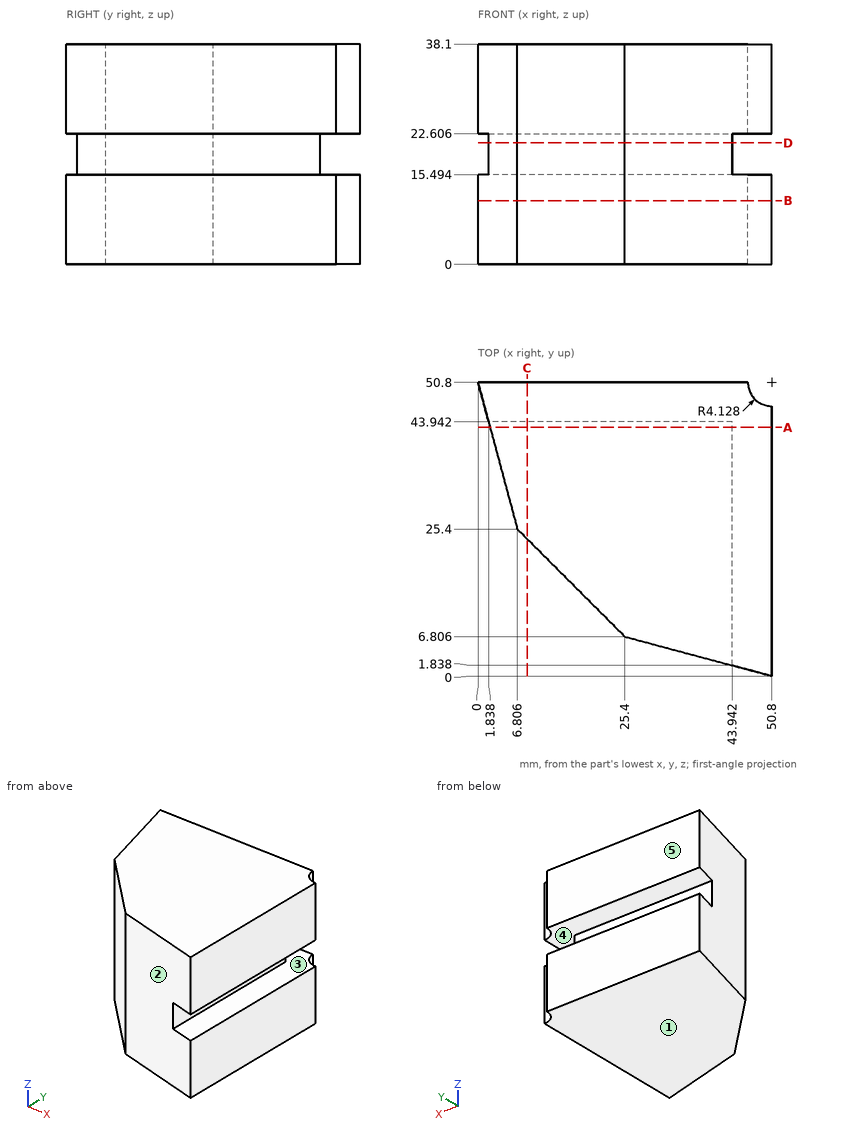
Job drawing, mm, ordinate dimensions from the low corner. One solid piece. A direction names the side the tool comes from. Round coordinates to 2 decimals unless told otherwise and drop trailing zeros. Loops run counter-clockwise (first coordinate to the right, second up) from the corner with the lowest first, then second, coordinate; pieces in that order, holes last. Notation, with made-up numbers: (13, 61) -> (21, 61) arc R11 ccw to (21, 76) -> close; hole circle Ø2 at (-15.75, 49). An arc over 180 degrees is marked (long way). Use CSV: the item, a comma, the result in double quotes. Start each with the question number.
Q1. Saw through at C-C on x = 8.5. Give the cut face in (y, z) (1 decimal).
Q2. Saw through at A-A on y = 43. Give the cut face in (x, z) (1 decimal).
Q3. Saw through at D-D on z = 21. Give the cut face in (x, y) (1 decimal).
Q4. Mould opens along Z. For the marked faces 1, 2 and 3 say: +Z half, -Z half, draft (parallel to the pull), parting line (faces both ways), or undercut.
Q5. Saw through at B-B on z = 11. Give the cut face in (x, y) (1 decimal), and give its area (3 significant figures).
Q6. Which spindle directions (+Z, -Z, +X, -X, +Y, -Y) get a long thin tool onto all of the face, cutting with end or side? Do the marked faces 4 and 5. Say none if no direction does.
Q7. Drill centre lines: L1, parallel to Z at x = 46, y = 40 (1 decimal); L2, parallel to X at y = 22, z = 2 (1 decimal). Where is each one in solid material? Low to high.
Q8. Flat gauge pins, fed straight in: pin 1 Ø3.5 at (x, z) = (21, 17.5) entering from +Y; pin 2 Ø1 at (y, z) = (23, 26) entering from -X (1 decimal); pin 3 Ø2 at (y, z) = (24.5, 20.5) entering from +X. Where does each tip first touch, or does it go through?
Solutions:
1,outline,"(23.7, 0) -> (50.8, 0) -> (50.8, 15.5) -> (43.9, 15.5) -> (43.9, 22.6) -> (50.8, 22.6) -> (50.8, 38.1) -> (23.7, 38.1) -> close"
2,outline,"(2.1, 0) -> (50.8, 0) -> (50.8, 15.5) -> (43.9, 15.5) -> (43.9, 22.6) -> (50.8, 22.6) -> (50.8, 38.1) -> (2.1, 38.1) -> close"
3,outline,"(1.8, 43.9) -> (6.8, 25.4) -> (25.4, 6.8) -> (43.9, 1.8) -> (43.9, 43.9) -> close"
4,face 1,"-Z half"
4,face 2,"draft"
4,face 3,"undercut"
5,outline,"(0, 50.8) -> (6.8, 25.4) -> (25.4, 6.8) -> (50.8, 0) -> (50.8, 46.7) arc R4.1 cw to (46.7, 50.8) -> close"
5,area,"1,920 mm^2"
6,face 4,"+X, +Y"
6,face 5,"+Z, -Z, +X, -X, +Y"
7,L1,"z = 0 to 15.5, 22.6 to 38.1"
7,L2,"x = 10.2 to 50.8"
8,pin 1,"stops at y = 43.94"
8,pin 2,"stops at x = 8.7"
8,pin 3,"stops at x = 43.94"
